from build123d import *

# Parameters (mm, degrees)
SKETCH_R  = 6.6
PAD_DEPTH = 8


with BuildPart() as part:
    # Sketch → Pad (new body)
    with BuildSketch(Plane.XY):
        with BuildLine():
            Line((-4, 40), (-146, 40))
            ThreePointArc((-146, 40), (-154.485281, 36.485281), (-158, 28))
            Line((-158, -55), (-158, 28))
            ThreePointArc((-188.565904, -97.622258), (-166.431336, -81.224661), (-158, -55))
            ThreePointArc((-188.565904, -97.622258), (-202.717412, -121.203739), (-181.74971, -139))
            Line((-181.74971, -139), (-4, -139))
            ThreePointArc((-4, -139), (-1.171573, -137.828427), (0, -135))
            Line((0, 36), (0, -135))
            ThreePointArc((0, 36), (-1.171573, 38.828427), (-4, 40))
        make_face()
        with Locations((-37, 25)):
            Circle(SKETCH_R, mode=Mode.SUBTRACT)
        with Locations((-37, -25)):
            Circle(SKETCH_R, mode=Mode.SUBTRACT)
        with Locations((-14, 13)):
            Circle(SKETCH_R, mode=Mode.SUBTRACT)
        with Locations((-14, -13)):
            Circle(SKETCH_R, mode=Mode.SUBTRACT)
        with Locations((-164, -126)):
            Circle(SKETCH_R, mode=Mode.SUBTRACT)
        with Locations((-114, -126)):
            Circle(SKETCH_R, mode=Mode.SUBTRACT)
        with Locations((-64, -126)):
            Circle(SKETCH_R, mode=Mode.SUBTRACT)
        with Locations((-90.2, -70)):
            Circle(SKETCH_R, mode=Mode.SUBTRACT)
        with BuildLine():
            Line((-40.101765, 6.2), (-33.898235, 6.2))
            ThreePointArc((-33.898235, 6.2), (-33.357039, 6.274615), (-32.856224, 6.492893))
            ThreePointArc((-30.107107, 3.743776), (-30.4, 6.2), (-32.856224, 6.492893))
            ThreePointArc((-30.107107, 3.743776), (-30.325385, 3.242961), (-30.4, 2.701765))
            Line((-30.4, 2.701765), (-30.4, -2.701765))
            ThreePointArc((-30.4, -2.701765), (-30.325385, -3.242961), (-30.107107, -3.743776))
            ThreePointArc((-32.856224, -6.492893), (-30.4, -6.2), (-30.107107, -3.743776))
            ThreePointArc((-32.856224, -6.492893), (-33.357039, -6.274615), (-33.898235, -6.2))
            Line((-33.898235, -6.2), (-40.101765, -6.2))
            ThreePointArc((-40.101765, -6.2), (-40.642961, -6.274615), (-41.143776, -6.492893))
            ThreePointArc((-43.892893, -3.743776), (-43.6, -6.2), (-41.143776, -6.492893))
            ThreePointArc((-43.892893, -3.743776), (-43.674615, -3.242961), (-43.6, -2.701765))
            Line((-43.6, -2.701765), (-43.6, 2.701765))
            ThreePointArc((-43.6, 2.701765), (-43.674615, 3.242961), (-43.892893, 3.743776))
            ThreePointArc((-41.143776, 6.492893), (-43.6, 6.2), (-43.892893, 3.743776))
            ThreePointArc((-41.143776, 6.492893), (-40.642961, 6.274615), (-40.101765, 6.2))
        make_face(mode=Mode.SUBTRACT)
        with BuildLine():
            Line((-90.7, 20.3), (-89.943823, 20.3))
            ThreePointArc((-89.943823, 20.3), (-88.049637, 20.561153), (-86.296785, 21.325126))
            ThreePointArc((-76.674874, 11.703215), (-77.700001, 20.3), (-86.296785, 21.325126))
            ThreePointArc((-76.674874, 11.703215), (-77.438847, 9.950364), (-77.7, 8.056178))
            Line((-77.7, 8.056178), (-77.7, -8.056178))
            ThreePointArc((-77.7, -8.056178), (-77.438847, -9.950365), (-76.674874, -11.703216))
            ThreePointArc((-86.296785, -21.325126), (-77.7, -20.3), (-76.674874, -11.703216))
            ThreePointArc((-86.296785, -21.325126), (-88.049636, -20.561153), (-89.943822, -20.3))
            Line((-90.7, -20.3), (-89.943822, -20.3))
            ThreePointArc((-96.2, -30.280093), (-90.502363, -26.91448), (-90.7, -20.3))
            Line((-96.2, -30.280093), (-120, -30.280093))
            ThreePointArc((-120, -27.280093), (-121.5, -28.780093), (-120, -30.280093))
            Line((-96.2, -27.280093), (-120, -27.280093))
            ThreePointArc((-96.2, -27.280093), (-92.20498, -23.080559), (-96.598572, -19.3))
            Line((-128.601428, -22.504808), (-96.598572, -19.3))
            ThreePointArc((-133, -18.524715), (-131.683814, -21.490713), (-128.601428, -22.504808))
            Line((-133, 18.524715), (-133, -18.524715))
            ThreePointArc((-128.601428, 22.504808), (-131.683814, 21.490713), (-133, 18.524715))
            Line((-128.601428, 22.504808), (-96.598572, 19.3))
            ThreePointArc((-96.598572, 19.3), (-92.20498, 23.080559), (-96.2, 27.280093))
            Line((-96.2, 27.280093), (-120, 27.280093))
            ThreePointArc((-120, 30.280093), (-121.5, 28.780093), (-120, 27.280093))
            Line((-96.2, 30.280093), (-120, 30.280093))
            ThreePointArc((-90.7, 20.3), (-90.502363, 26.91448), (-96.2, 30.280093))
        make_face(mode=Mode.SUBTRACT)
    extrude(amount=-PAD_DEPTH)


solid = part.part
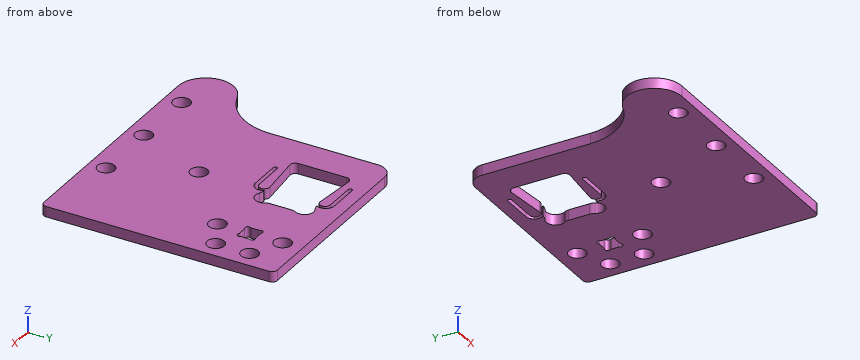
Can you work these out from the model? Positions are in its coordinate system, mm. Coordinates: 2 decimals unless noted, no trailing zeros. Loops run counter-clockwise (first coordinate to the right, second up) from the corner with the lowest first, then second, coordinate; pieces in that order, holes last. Notation, with made-up numbers: M 72,71 L 94,71 A4 ccw 94,77 Z; hole C 79.25,29 d9. An arc over 180 degrees is marked long. Return JSON: item names as keys, results as strings. Group by question number.
Item 1: I'm going to push flat-ended pins straight in: pin 1 Ø4 at (y, z) = (3, -3) entering from -X; pin 2 Ø4 at (y, z) = (-70, -2) entering from -X. Where does each tip first touch, or does it pass through?
Item 2: Imagine slicing it at A-A (x = -14). Please give me the cut outline in (y, z).
Item 3: If I drill on L1, parallel to Y at x = -37, z = -7.5; L2, parallel to Y at x = -99.5, z = -5.25; L3, parallel to Y at x = -14, z = -4, over which ranges is the centre line in solid material (lowest first)? Write a range as from..to.
Item 4: Imagine slicing it at C-C (y = -70). Please give me the cut outline in (x, z).
Item 5: Imagine slicing it at B-B (x = -61). Please give me the cut outline in (y, z), and give its area (3 significant figures).
Item 6: Imagine slicing it at D-D (x = -37). Please give me the cut outline in (y, z).
Verdict:
{
 "1": {"pin 1": "stops at x = -158", "pin 2": "stops at x = -161.33"},
 "2": {"outline": "M -139,-8 L -19.6,-8 L -19.6,0 L -139,0 Z; M -6.4,-8 L 6.4,-8 L 6.4,0 L -6.4,0 Z; M 19.6,-8 L 40,-8 L 40,0 L 19.6,0 Z"},
 "3": {"L1": "y = -139..-31.6, -18.4..-6.2, 6.2..18.4, 31.6..40", "L2": "y = -139..-30.28, -27.28..-19.59, 19.59..27.28, 30.28..40", "L3": "y = -139..-19.6, -6.4..6.4, 19.6..40"},
 "4": {"outline": "M -160.57,-8 L -96.8,-8 L -96.8,0 L -160.57,0 Z; M -83.6,-8 L 0,-8 L 0,0 L -83.6,0 Z"},
 "5": {"outline": "M -139,-8 L -131.88,-8 L -131.88,0 L -139,0 Z; M -120.12,-8 L 40,-8 L 40,0 L -120.12,0 Z", "area": "1,340 mm^2"},
 "6": {"outline": "M -139,-8 L -31.6,-8 L -31.6,0 L -139,0 Z; M -18.4,-8 L -6.2,-8 L -6.2,0 L -18.4,0 Z; M 6.2,-8 L 18.4,-8 L 18.4,0 L 6.2,0 Z; M 31.6,-8 L 40,-8 L 40,0 L 31.6,0 Z"}
}
